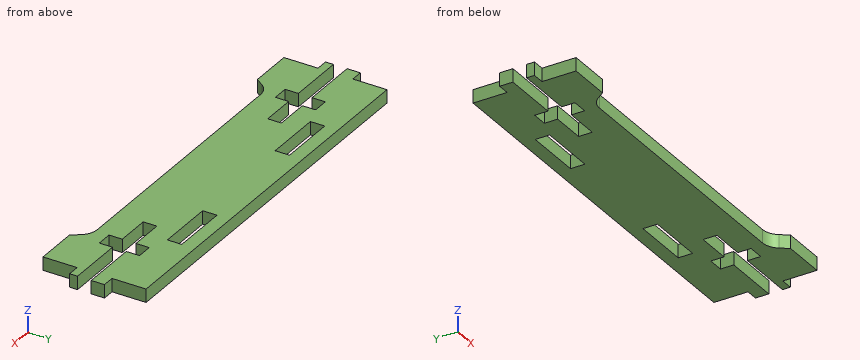
```python
from build123d import *

# Parameters (mm, degrees)
BOSS_EXTRUDE1_DEPTH = 3.7
FILLET1_R           = 5
SKETCH3_W           = 16
SKETCH3_H           = 4
CUT_EXTRUDE1_DEPTH  = 62.374947331


with BuildPart() as part:
    # Sketch2 → Boss-Extrude1 (new body)
    with BuildSketch(Plane.XY):
        Polygon((-54.64, 19.610011726), (54.64, 19.610011726), (54.64, 10.110011726), (58.04, 10.110011726), (58.04, 6.410011726), (42.14, 6.410011726), (42.14, 10.110011726), (37.74, 10.110011726), (37.74, 6.410011726), (28.24, 6.410011726), (28.24, 2.610011726), (37.74, 2.610011726), (37.74, -1.089988274), (42.14, -1.089988274), (42.14, 2.610011726), (58.04, 2.610011726), (58.04, 0.410011726), (54.64, 0.410011726), (54.64, -9.089988274), (42.64, -9.089988274), (39.572296355, -4.769343347), (-39.572296355, -4.769343347), (-42.64, -9.089988274), (-54.64, -9.089988274), (-54.64, 0.410011726), (-58.04, 0.410011726), (-58.04, 2.610011726), (-42.14, 2.610011726), (-42.14, -1.089988274), (-37.74, -1.089988274), (-37.74, 2.610011726), (-28.24, 2.610011726), (-28.24, 6.410011726), (-37.74, 6.410011726), (-37.74, 10.110011726), (-42.14, 10.110011726), (-42.14, 6.410011726), (-58.04, 6.410011726), (-58.04, 10.110011726), (-54.64, 10.110011726), align=None)
    extrude(amount=BOSS_EXTRUDE1_DEPTH)

    # Fillet1
    fillet1_edges = [part.edges().sort_by_distance(p)[0] for p in [
        (39.572296355, -4.769343347, 1.85),
        (-39.572296355, -4.769343347, 1.85),
    ]]
    fillet(fillet1_edges, radius=FILLET1_R)

    # Sketch3 → Cut-Extrude1 (cut, through all)
    with BuildSketch(Plane.XY.offset(3.7)):
        with Locations((24.44, 13.910011726)):
            Rectangle(SKETCH3_W, SKETCH3_H)
        with Locations((-24.44, 13.910011726)):
            Rectangle(SKETCH3_W, SKETCH3_H)
    extrude(amount=-CUT_EXTRUDE1_DEPTH, mode=Mode.SUBTRACT)


solid = part.part
```
Geometry check sheet. Reference: the model listing, model coordinates, mm. Coordinates: 2 decimals unless noted, no trailing zeros. Order: outer loops, then holes, each group sorted by start corner. A loop starts at its lowest first (then second) coordinate and runs counter-clockwise, first axis right, second up. Notation, with made-up numbers: (2.25, 56.5) - (31.25, 56.5) arc R32 cw to (31.25, 85.5) - close; hole circle Ø2 at (89.25, -28.75). An arc over 180 degrees is marked (long way). Answer as a JSON object with one key per item and string values. Group by question number.
Item 1: Sectioned sample at B-B, the plane z = 1.55. Give the number of separate pieces and of enclosed holes in the cut face, and give its area (3 significant figures).
Item 2: Sectioned sample at A-A, the plane x = -51. Record the cut outline in (y, z).
Item 3: Scan lines: probe 1 along X at (y, z) = (12.5, 3.1); probe 2 along X at (y, z) = (-0.5, 2.85); probe 3 along Y at (x, z) = (-30, 0.7). Record each from-to range of solid material in increasing order.
Item 4: Sectioned sample at C-C, the plane x = 10.5. Record the cut outline in (y, z).
Item 5: Depth check by flat-ended pin: pin 1 Ø1.1 at (y, z) = (13, 2) entering from +X; pin 2 Ø1.5 at (y, z) = (4, 2) entering from -X; pin 3 Ø1.1 at (x, z) = (32, 2) entering from -Y. Enter the tip coordinate at first touch or a pass-through.
Resolved:
{
 "1": {"separate pieces": "1", "enclosed holes": "2", "area": "2,430 mm^2"},
 "2": {"outline": "(-9.09, 0) - (2.61, 0) - (2.61, 3.7) - (-9.09, 3.7) - close; (6.41, 0) - (19.61, 0) - (19.61, 3.7) - (6.41, 3.7) - close"},
 "3": {"probe 1": "-54.64 to -32.44, -16.44 to 16.44, 32.44 to 54.64", "probe 2": "-54.64 to -42.14, -37.74 to 37.74, 42.14 to 54.64", "probe 3": "-4.77 to 2.61, 6.41 to 11.91, 15.91 to 19.61"},
 "4": {"outline": "(-4.77, 0) - (19.61, 0) - (19.61, 3.7) - (-4.77, 3.7) - close"},
 "5": {"pin 1": "x = 54.64", "pin 2": "x = -28.24", "pin 3": "y = -4.77"}
}
